Job drawing, mm, ordinate dimensions from the low corner. One solid piece. A direction names the side the tool comes from. Give positions to 0.01 mm unless a question says otherwise; leave off trailing zeros. Write each loop counter-clockwise with the first axis right and the second up, starting at its lowest first coordinate (ties: lowest second). Pieces come first, ordered by that corner, then holes. Notation, with made-up numbers: M 36,-35.5 L 79,-35.5 A20 cw 79,-24.5 Z; hole C 81.25,60 d5. An arc over 180 degrees is marked long. Use a Markdown table: item, result.
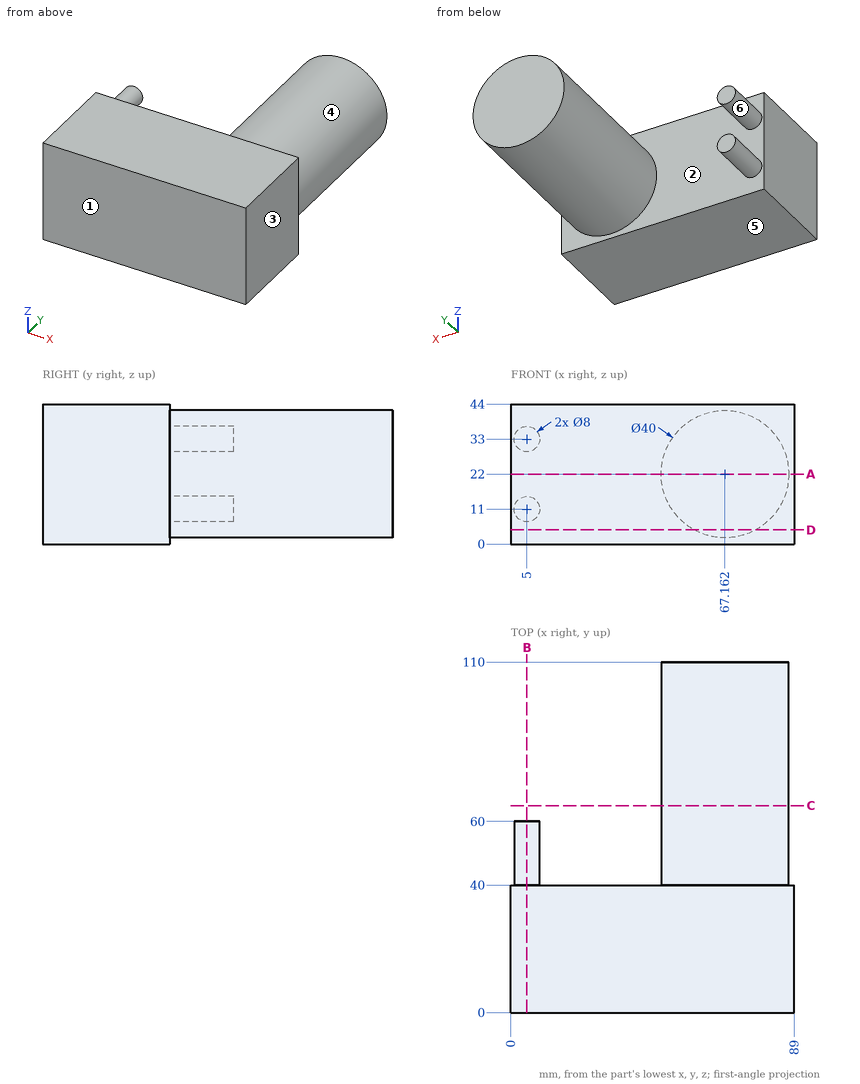
1. Two-plate mould, pull along Z, no slides. Class the marked faces 3, 4, 5 and 6: released by +Z, released by -Z, zero draft, split by the parting line, or undercut.
Findings below:
| item | result |
|---|---|
| face 3 | zero draft |
| face 4 | split by the parting line |
| face 5 | released by -Z |
| face 6 | undercut |
2. Cut at A-A, the plane z = 22. Give the cut face in (x, y), then the cut area to 3 significant figures.
Findings below:
| item | result |
|---|---|
| outline | M 0,0 L 89,0 L 89,40 L 87.16,40 L 87.16,110 L 47.16,110 L 47.16,40 L 0,40 Z |
| area | 6,360 mm2 |
3. Cut at D-D, the plane z = 4.5. Give the cut face in (x, y) (1 decimal), then the cut area to 3 significant figures.
Findings below:
| item | result |
|---|---|
| outline | M 0,0 L 89,0 L 89,40 L 76.8,40 L 76.8,110 L 57.5,110 L 57.5,40 L 0,40 Z |
| area | 4,920 mm2 |
4. Drill centre lines: L1, parallel to Y at x = 4.5, z = 7; L2, parallel to Z at x = 57.5, y = 61.5; L3, parallel to X at y = 92.5, z = 27.5 (1 decimal). Where is each one in solid material? Low to high.
Findings below:
| item | result |
|---|---|
| L1 | 0 to 40 |
| L2 | 4.49 to 39.51 |
| L3 | 47.9 to 86.4 |
5. Cut at C-C, the plane y = 65. Give the cut face in (x, z).
Findings below:
| item | result |
|---|---|
| outline | C 67.16,22 d40 |
6. Cut at B-B, the plane x = 5. Give the cut face in (y, z).
Findings below:
| item | result |
|---|---|
| outline | M 0,0 L 40,0 L 40,7 L 60,7 L 60,15 L 40,15 L 40,29 L 60,29 L 60,37 L 40,37 L 40,44 L 0,44 Z |
7. Drop flat-ended pins along their axis: P1, Ø9, axis at x = 7, z = 32.5, coming from the +Y side; P2, Ø2, axis at y = 68, z = 7.5, coming from the +X side; P3, Ø10, axis at x = 39.5, y = 82, coming from the +Z side; P4, Ø12, axis at y = 71.5, z = 4.5, coming from the -X side. Give the stop position or say it passes through.
Findings below:
| item | result |
|---|---|
| P1 | y = 60 |
| P2 | x = 81.92 |
| P3 | through |
| P4 | x = 50.8 |
8. Tool access for the marked faces 1 and 2: list every direction of +Z, -Z, +X, -X, +Y, -Y with a clear straight run to the whole face (end or side of a thin tool).
Findings below:
| item | result |
|---|---|
| face 1 | +Z, -Z, +X, -X, -Y |
| face 2 | +Y |
